```python
from build123d import *

# Parameters (mm, degrees)
SKETCH1_W           = 8.5
SKETCH1_H           = 8.5
SKETCH1_R           = 1.5
BOSS_EXTRUDE1_DEPTH = 19.5
CHAMFER1_SIZE       = 0.5


with BuildPart() as part:
    # Sketch1 → Boss-Extrude1 (new body)
    with BuildSketch(Plane(origin=(0, 0, 0), x_dir=(1, 0, 0), z_dir=(0, 1, 0))):
        Rectangle(SKETCH1_W, SKETCH1_H)
        with Locations(Location((0, 0, 0), (0, 0, 270))):
            Circle(SKETCH1_R, mode=Mode.SUBTRACT)
    extrude(amount=BOSS_EXTRUDE1_DEPTH)

    # Chamfer1
    chamfer1_edges = [part.edges().sort_by_distance(p)[0] for p in [
        (-4.25, 19.5, 0),
        (0, 19.5, 4.25),
        (4.25, 19.5, 0),
        (0, 0, 4.25),
        (-4.25, 0, 0),
        (0, 0, -4.25),
        (4.25, 0, 0),
        (4.25, 9.75, 4.25),
        (-4.25, 9.75, 4.25),
        (-4.25, 9.75, -4.25),
        (4.25, 9.75, -4.25),
        (0, 19.5, -4.25),
    ]]
    chamfer(chamfer1_edges, length=CHAMFER1_SIZE)


solid = part.part
```
CAD build for the part. Positions are in the model's coordinates, mm. Round coordinates to 2 decimals unless told otherwise and drop trailing zeros. Loops run counter-clockwise (first coordinate to the right, second up) from the corner with the lowest first, then second, coordinate; pieces in that order, holes last. Notation, with made-up numbers: (57.5, 12.25) - (73.5, 12.25) arc R22 cw to (73.5, 26.25) - close; hole circle Ø11 at (56, -13.75). An arc over 180 degrees is marked (long way). Return JSON: item names as keys, results as strings. Group by question number.
Q1. Band-saw the part on C-C on x = 0. Give the cut face in (y, z), plus the area to 3 significant figures.
Q2. Drill centre lines: line 1 along X through (y, z) = (15, 0); line 2 along Z through (x, y) = (0.75, 17.25). Where is each one in solid material? Low to high. Write a range as [from, to].
Q3. Band-saw the part on B-B on y = 15.75. Give the cut face in (x, z).
Q4. Band-saw the part on A-A on z = 0. Give the cut face in (x, y).
Q5. Two-plate mould, pull along X, no slides. Class faces 1 (the face through (-4.25, 10, 0)), 2 (the face through (-2, 0, 0)), 3 (the face through (0.45, 9.61, 1.43)): +X half, -X half, draft (parallel to the pull), parting line (faces both ways), or undercut.
Solutions:
{
 "1": {"outline": "(0, -3.75) - (0.5, -4.25) - (19, -4.25) - (19.5, -3.75) - (19.5, -1.5) - (0, -1.5) - close; (0, 1.5) - (19.5, 1.5) - (19.5, 3.75) - (19, 4.25) - (0.5, 4.25) - (0, 3.75) - close", "area": "107 mm^2"},
 "2": {"line 1": "x = [-4.25, -1.5], [1.5, 4.25]", "line 2": "z = [-4.25, -1.3], [1.3, 4.25]"},
 "3": {"outline": "(-4.25, -3.75) - (-3.75, -4.25) - (3.75, -4.25) - (4.25, -3.75) - (4.25, 3.75) - (3.75, 4.25) - (-3.75, 4.25) - (-4.25, 3.75) - close; hole circle Ø3 at (0, 0)"},
 "4": {"outline": "(-4.25, 0.5) - (-3.75, 0) - (-1.5, 0) - (-1.5, 19.5) - (-3.75, 19.5) - (-4.25, 19) - close; (1.5, 0) - (3.75, 0) - (4.25, 0.5) - (4.25, 19) - (3.75, 19.5) - (1.5, 19.5) - close"},
 "5": {"face 1": "-X half", "face 2": "draft", "face 3": "undercut"}
}
